Autodesk Inventor part; units mm, degrees
ref_plane "YZ Plane" through (0, 0, 0) normal (1, 0, 0) x (0, 1, 0)
ref_plane "XZ Plane" through (0, 0, 0) normal (0, 1, 0) x (-1, 0, 0)
ref_plane "XY Plane" through (0, 0, 0) normal (0, 0, 1) x (1, 0, 0)
sketch "Sketch1" plane through (0, 0, 0) normal (0, 0, 1) x (1, 0, 0)
  line L0 (-19, 19) -> (19, 19)
  line L1 (19, 19) -> (19, -19)
  line L2 (19, -19) -> (-19, -19)
  line L3 (-19, -19) -> (-19, 19)
  line L4 (-19, 19) -> (19, -19) construction
  line L5 (19, 19) -> (-19, -19) construction
  line L6 (-11, 11) -> (11, -11) construction
  line L7 (11, 11) -> (-11, -11) construction
  circle A0 centre (0, 0) radius 13.5
  dimension "d0" = 38
  dimension "d1" = 38
  dimension "d2" = 22
  dimension "d3" = 22
  dimension "d30" = 27
extrude "Extrusion1" add sketch "Sketch1" along normal mid plane 2
sketch "Sketch2" plane through (0, 0, 1) normal (0, 0, 1) x (1, 0, 0)
  line L0 (-13, 13) -> (13, -13) construction
  line L1 (13, 13) -> (-13, -13) construction
  line L2 (-11.5, -11.5) -> (11.5, 11.5) construction
  line L3 (11.5, -11.5) -> (-11.5, 11.5) construction
  circle A0 centre (0, 0) radius 13.5
  circle A1 centre (0, 0) radius 14.5
  dimension "d6" = 26
  dimension "d7" = 26
  dimension "d8" = 23
  dimension "d28" = 27
  dimension "d29" = 29
extrude "Extrusion2" add sketch "Sketch2" along normal blind 33
sketch "Sketch3" plane through (0, 0, -1) normal (0, 0, -1) x (-1, 0, 0)
  line L0 (19, 19) -> (19, -19)
  line L1 (19, -19) -> (-19, -19)
  line L2 (-19, -19) -> (-19, 19)
  line L3 (-19, 19) -> (19, 19)
  circle A0 centre (0, 0) radius 13.5
  point P0 (15, -15)
  point P1 (-15, -15)
  point P2 (15, 15)
  point P3 (-15, 15)
  dimension "d11" = 15
  dimension "d12" = 15
  dimension "d15" = 30
  dimension "d18" = 30
hole "Hole1" at (-15, -15, -1) at (15, -15, -1) at (-15, 15, -1) at (15, 15, -1) direction (0, 0, 1) diameter 3.4 end through all
equation "\"d1\" = d0"
equation "\"d3\" = d2"
equation "\"d7\" = d6"
properties part number "tube"
Verification items for the finished model (mm, model axes). A direction names the side the tool comes from. Round coordinates to 2 decimals unless told otherwise and drop trailing zeros. Order: outer loops, then holes, each group sorted by start corner. A loop starts at its lowest first (then second) coordinate and runs counter-clockwise, first axis right, second up.
1. Section check C-C on z = 2. Record the cut outline in (x, y), then the cut area to 3 significant figures.
Final values:
outline: circle Ø29 at (0, 0); hole circle Ø27 at (0, 0)
area: 88.0 mm2
2. Go/stop test with flat-tipped pins: P1, Ø2, axis at y = -9.5, z = 5.5, coming from the +X side; P2, Ø1, axis at y = -1.5, z = 20.5, coming from the +X side; P3, Ø4, axis at x = 15, y = 15, coming from the -Z side; P4, Ø4, axis at x = -15, y = -15, coming from the +Z side. Record where each tip stops, or that it passes through.
Final values:
P1: stops at x = 11.75
P2: stops at x = 14.47
P3: stops at z = -1
P4: stops at z = 1
3. Thickness scan on L1, parallel to Y at x = 15, z = 0; L2, parallel to Z at x = 11, y = 17.5. Record the ranges inside material, lowest first.
Final values:
L1: y = -19 to -16.7, -13.3 to 13.3, 16.7 to 19
L2: z = -1 to 1
4. Section check A-A on x = 0. Record the cut outline in (y, z).
Final values:
outline: (-19, -1) - (-13.5, -1) - (-13.5, 34) - (-14.5, 34) - (-14.5, 1) - (-19, 1) - close; (13.5, -1) - (19, -1) - (19, 1) - (14.5, 1) - (14.5, 34) - (13.5, 34) - close
5. Release check for a two-part mould opening along X. For faces 3 (the cylindrical face through (6.691, 12.864, 17.269)), 4 (the flat face through (-12.9, 4.5, -1)), 5 (the cylindrical face through (-14.35, -13.43, 0.01)) record: +X half, -X half, draft (parallel to the pull), parting line (faces both ways), or undercut.
Final values:
face 3: parting line
face 4: draft
face 5: undercut
6. Access from +Z, -Z, +X, -X, +Y, -Y to the whole of each face (thin tool, end or side, straight path). Record for faces 1 (the flat face through (0, 19, 0)), 2 (the flat face through (-9, 13, 1)).
Final values:
face 1: +Z, -Z, +X, -X, +Y
face 2: +Z
